Check sheet for the modelled part. Datum: model origin and axes. Units: mm. A direction names the side the tool comes from. Round coordinates to 2 decimals unless told otherwise and drop trailing zeros. Write each loop counter-clockwise with the first axis right and the second up, starting at its lowest first coordinate (ties: lowest second). Pieces come first, ordered by that corner, then holes. Notation, with made-up numbers: (73, -37) -> (120, -37) arc R20 cw to (120, -12) -> close; hole circle Ø2 at (25.5, 73.25). An arc over 180 degrees is marked (long way). One line per item, written item: value. Start each with the question number.
Autodesk Inventor part; units mm, degrees
ref_plane "YZ Plane" through (0, 0, 0) normal (1, 0, 0) x (0, 1, 0)
ref_plane "XZ Plane" through (0, 0, 0) normal (0, 1, 0) x (-1, 0, 0)
ref_plane "XY Plane" through (0, 0, 0) normal (0, 0, 1) x (1, 0, 0)
sketch "Sketch1" plane through (0, 0, 0) normal (0, 0, 1) x (1, 0, 0)
  line L0 (0, 0) -> (132, 0)
  line L1 (132, 0) -> (132, 98)
  line L2 (132, 98) -> (0, 98)
  line L3 (0, 98) -> (0, 0)
  line L4 (16, 101) -> (26, 101)
  line L5 (26, 101) -> (26, -3)
  line L6 (26, -3) -> (16, -3)
  line L7 (16, -3) -> (16, 101)
  line L8 (102, 101) -> (92, 101)
  line L9 (92, 101) -> (92, -3)
  line L10 (92, -3) -> (102, -3)
  line L11 (102, -3) -> (102, 101)
  line L12 (0, 88) -> (-3, 88)
  line L13 (-3, 88) -> (-3, 78)
  line L14 (-3, 78) -> (0, 78)
  line L15 (0, 78) -> (0, 88)
  line L16 (0, 10) -> (-3, 10)
  line L17 (-3, 10) -> (-3, 20)
  line L18 (-3, 20) -> (0, 20)
  line L19 (0, 20) -> (0, 10)
  line L20 (0, 54) -> (-3, 54)
  line L21 (-3, 54) -> (-3, 44)
  line L22 (-3, 44) -> (0, 44)
  line L23 (0, 44) -> (0, 54)
  line L24 (0, 98) -> (9, 98)
  line L25 (9, 98) -> (9, 93)
  line L26 (8, 92) -> (0, 92)
  line L27 (0, 92) -> (0, 98)
  arc A0 (8, 92) -> (9, 93) centre (8, 93) ccw
  point P0 (9, 92)
  dimension "d0" = 98
  dimension "d1" = 132
  dimension "d74" = 10
  dimension "d77" = 10
  dimension "d306" = 16
  dimension "d307" = 104
  dimension "d308" = 3
  dimension "d309" = 3
  dimension "d310" = 104
  dimension "d311" = 30
  dimension "d312" = 3
  dimension "d313" = 10
  dimension "d314" = 10
  dimension "d315" = 3
  dimension "d316" = 10
  dimension "d317" = 10
  dimension "d318" = 10
  dimension "d319" = 3
  dimension "d320" = 24
  dimension "d368" = 9
  dimension "d369" = 6
  dimension "d370" = 1
extrude "Extrusion1" add sketch "Sketch1" along normal blind 3 contours L3 L26 A0 L25 L2 L7 L0 | L7 L2 L5 L0 | L0 L5 L6 L7 | L16 L17 L18 L3 | L5 L2 L9 L0 | L7 L4 L5 L2 | L9 L2 L11 L0 | L0 L11 L10 L9 | L22 L21 L20 L3 | L11 L2 L1 L0 | L9 L8 L11 L2 | L14 L13 L12 L3
sketch "Sketch11" plane through (0, 0, 3) normal (0, 0, 1) x (1, 0, 0)
  line L0 (0, 0) -> (0, 98)
  line L1 (6, 0) -> (0, 0)
  point P0 (15, 20.5)
  dimension "d141" = 20.5
  dimension "d142" = 15
hole "Hole7" at (15, 20.5, 3) direction (0, 0, -1) diameter 22 end through all
sketch "Sketch12" plane through (0, 0, 3) normal (0, 0, 1) x (1, 0, 0)
  circle A0 centre (15, 20.5) radius 11
  point P0 (3.5, 32)
  point P1 (26.5, 9)
  point P2 (3.5, 9)
  dimension "d152" = 11.5
  dimension "d153" = 11.5
  dimension "d161" = 11.5
  dimension "d162" = 11.5
  dimension "d163" = 11.5
  dimension "d164" = 11.5
hole "Hole8" at (3.5, 32, 3) at (26.5, 9, 3) at (3.5, 9, 3) direction (0, 0, -1) diameter 2.5 end through all
sketch "Sketch20" plane through (0, 0, 3) normal (0, 0, 1) x (1, 0, 0)
  line L0 (132, 0) -> (120, 0)
  line L1 (132, 98) -> (132, 0)
  line L2 (120, 98) -> (132, 98)
  line L3 (125.5, 73.7) -> (128, 73.7)
  line L4 (128, 73.7) -> (128, 72.3)
  line L5 (128, 72.3) -> (125.5, 72.3)
  line L6 (125.5, 72.3) -> (125.5, 73.7)
  line L7 (125.5, 63.7) -> (128, 63.7)
  line L8 (128, 63.7) -> (128, 62.3)
  line L9 (128, 62.3) -> (125.5, 62.3)
  line L10 (125.5, 62.3) -> (125.5, 63.7)
  line L11 (125.5, 13.7) -> (128, 13.7)
  line L12 (128, 13.7) -> (128, 12.3)
  line L13 (128, 12.3) -> (125.5, 12.3)
  line L14 (125.5, 12.3) -> (125.5, 13.7)
  line L15 (125.5, 3.7) -> (128, 3.7)
  line L16 (128, 3.7) -> (128, 2.3)
  line L17 (128, 2.3) -> (125.5, 2.3)
  line L18 (125.5, 2.3) -> (125.5, 3.7)
  dimension "d208" = 1.4
  dimension "d209" = 24.3
  dimension "d210" = 4
  dimension "d211" = 2.5
  dimension "d212" = 1.4
  dimension "d213" = 8.6
  dimension "d214" = 2.5
  dimension "d215" = 1.4
  dimension "d216" = 2.3
  dimension "d217" = 4
  dimension "d218" = 8.6
  dimension "d219" = 1.4
extrude "Extrusion10" cut sketch "Sketch20" against normal through all
sketch "Sketch26" plane through (0, 0, 3) normal (0, 0, 1) x (1, 0, 0)
  line L0 (0, 98) -> (6, 98)
  line L1 (0, 88) -> (0, 98)
  point P0 (17, 85.25)
  point P1 (17, 78.75)
  dimension "d289" = 6.5
  dimension "d290" = 12.75
  dimension "d366" = 17
hole "Hole13" at (17, 85.25, 3) at (17, 78.75, 3) direction (0, 0, -1) diameter 2 end through all
sketch "草圖28" plane through (0, 0, 3) normal (0, 0, 1) x (1, 0, 0)
  line L0 (132, 0) -> (102, 0)
  line L1 (132, 98) -> (132, 0)
  line L2 (102, 98) -> (132, 98)
  line L3 (110.5, 98) -> (113.5, 98)
  line L4 (113.5, 98) -> (113.5, 89)
  line L5 (113.5, 89) -> (110.5, 89)
  line L6 (110.5, 89) -> (110.5, 98)
  line L7 (109.25, 89) -> (114.75, 89)
  line L8 (114.75, 89) -> (114.75, 91.3)
  line L9 (114.75, 91.3) -> (109.25, 91.3)
  line L10 (109.25, 91.3) -> (109.25, 89)
  line L11 (113.5, 9) -> (110.5, 9)
  line L12 (110.5, 9) -> (110.5, 0)
  line L13 (110.5, 0) -> (113.5, 0)
  line L14 (113.5, 0) -> (113.5, 9)
  line L15 (109.25, 9) -> (114.75, 9)
  line L16 (114.75, 9) -> (114.75, 6.7)
  line L17 (114.75, 6.7) -> (109.25, 6.7)
  line L18 (109.25, 6.7) -> (109.25, 9)
  dimension "d321" = 9
  dimension "d323" = 3
  dimension "d324" = 5.5
  dimension "d325" = 2.3
  dimension "d326" = 1.25
  dimension "d327" = 18.5
  dimension "d328" = 18.5
  dimension "d329" = 9
  dimension "d330" = 5.5
  dimension "d331" = 2.3
  dimension "d378" = 1.25
extrude "擠出14" cut sketch "草圖28" against normal through all
sketch "草圖29" plane through (0, 0, 3) normal (0, 0, 1) x (1, 0, 0)
  line L0 (26, 98) -> (16, 98)
  line L1 (0, 54) -> (0, 78)
  point P0 (0, 98)
  point P1 (8, 49)
  dimension "d336" = 8
  dimension "d337" = 49
hole "孔14" at (8, 49, 3) direction (0, 0, -1) diameter 3.5 end through all
sketch "草圖30" plane through (0, 0, 3) normal (0, 0, 1) x (1, 0, 0)
  circle A0 centre (8, 49) radius 1.75
  line L0 (132, 0) -> (113.5, 0)
  line L1 (132, 98) -> (132, 0)
  line L2 (113.5, 98) -> (132, 98)
  point P0 (8, 55)
  point P1 (8, 43)
  point P2 (120, 21.5)
  point P3 (126, 38.5)
  point P4 (127, 55)
  point P5 (127, 88)
  dimension "d345" = 6
  dimension "d346" = 6
  dimension "d371" = 21.5
  dimension "d372" = 12
  dimension "d373" = 6
  dimension "d374" = 38.5
  dimension "d375" = 5
  dimension "d376" = 55
  dimension "d377" = 10
  dimension "d381" = 5
hole "孔15" at (8, 55, 3) at (8, 43, 3) at (127, 88, 3) at (127, 55, 3) at (126, 38.5, 3) at (120, 21.5, 3) direction (0, 0, -1) diameter 3 end through all
sketch "草圖31" plane through (0, 0, 3) normal (0, 0, 1) x (1, 0, 0)
  line L0 (26, 98) -> (92, 98)
  line L1 (0, 54) -> (0, 78)
  line L2 (18, 65) -> (117, 65)
  line L3 (110, 29.25) -> (18, 29.25)
  line L4 (18, 29.25) -> (18, 52.4223)
  arc A0 (18, 65) -> (15.6316, 56.6737) centre (18, 60.5) ccw
  arc A1 (118.3333, 39.5719) -> (122, 56.1414) centre (115, 49) ccw
  line L5 (115, 34.25) -> (115, 34.8579)
  line L6 (122, 60) -> (122, 56.1414)
  arc A2 (18, 52.4223) -> (15.6316, 56.6737) centre (13, 52.4223) ccw
  arc A3 (122, 60) -> (117, 65) centre (117, 60) ccw
  arc A4 (118.3333, 39.5719) -> (115, 34.8579) centre (120, 34.8579) ccw
  arc A5 (110, 29.25) -> (115, 34.25) centre (110, 34.25) ccw
  line L7 (132, 98) -> (132, 0)
  point P0 (115, 39)
  point P1 (18, 56)
  point P2 (132, 86.882)
  dimension "d354" = 35.75
  dimension "d356" = 33
  dimension "d358" = 18
  dimension "d359" = 9
  dimension "d360" = 20
  dimension "d362" = 5
  dimension "d379" = 10
  dimension "d380" = 17
extrude "擠出15" cut sketch "草圖31" against normal through all
fillet "圓角9" radius 5 2 edges at (18, 31.083, 1.5) (21.6661, 29.25, 1.5)
properties part number "plastic_part_52"
1. Release check for a two-part mould opening along Y. For faces 1 (the face through (125.735, 87.194, 1.479)), 2 (the face through (113.5, 95, 2)), 3 (the face through (-1, 88, 1)) record: +Y half, -Y half, draft (parallel to the pull), parting line (faces both ways), or undercut.
2. Cross-section at B-B (y = 21.5). Record the cut outline in (x, z).
3. Cross-section at C-C (x = 120). Record the cut outline in (y, z).
4. Depth check by flat-ended pin: pin 1 Ø0.9 at (y, z) = (100, 2) entering from -X; pin 2 Ø0.9 at (x, z) = (11.5, 1.5) entering from +Y; pin 3 Ø1.1 at (y, z) = (3, 1) entering from -X. Enter the tip coordinate at first touch or a pass-through.
5. Cross-section at A-A (x = 53.5). Record the cut outline in (y, z).
6. Cross-section at D-D (x = 94). Record the cut outline in (y, z).
7. Material ranges on probe 1 along X at (y, z) = (94, 1.2); probe 2 along Y at (x, z) = (82, 1.5); probe 3 along X at (y, z) = (8.5, 1), recorded low to high.
8. Access from +Z, -Z, +X, -X, +Y, -Y to the whole of each face (thin tool, end or side, straight path). Record for faces 4 (the face through (-2, 20, 1)), 5 (the face through (26.587, 27.294, 1.479)), 6 (the face through (123, 98, 1)).
Working result:
1. face 1: undercut
1. face 2: draft
1. face 3: +Y half
2. outline: (0, 0) -> (4.05, 0) -> (4.05, 3) -> (0, 3) -> close; (25.95, 0) -> (118.5, 0) -> (118.5, 3) -> (25.95, 3) -> close; (121.5, 0) -> (132, 0) -> (132, 3) -> (121.5, 3) -> close
3. outline: (0, 0) -> (20, 0) -> (20, 3) -> (0, 3) -> close; (23, 0) -> (40.34, 0) -> (40.34, 3) -> (23, 3) -> close; (64, 0) -> (98, 0) -> (98, 3) -> (64, 3) -> close
4. pin 1: stops at x = 16
4. pin 2: stops at y = 98
4. pin 3: stops at x = 0
5. outline: (0, 0) -> (29.25, 0) -> (29.25, 3) -> (0, 3) -> close; (65, 0) -> (98, 0) -> (98, 3) -> (65, 3) -> close
6. outline: (-3, 0) -> (29.25, 0) -> (29.25, 3) -> (-3, 3) -> close; (65, 0) -> (101, 0) -> (101, 3) -> (65, 3) -> close
7. probe 1: x = 9 to 110.5, 113.5 to 132
7. probe 2: y = 0 to 29.25, 65 to 98
7. probe 3: x = 0 to 2.35, 4.65 to 25.35, 27.65 to 109.25, 114.75 to 132
8. face 4: +Z, -Z, -X
8. face 5: +Z, -Z
8. face 6: +Z, -Z, +X, +Y
